from build123d import *

# Parameters (mm, degrees)
PAD_DEPTH       = 25
SKETCH001_R     = 4.3
POCKET_DEPTH    = 20.501
SKETCH002_R     = 6.75
POCKET001_DEPTH = 15.501
FILLET_R        = 4
FILLET001_R     = 18


with BuildPart() as part:
    # Sketch → Pad (new body)
    with BuildSketch(Plane.XZ):
        with BuildLine():
            Line((40.4, -20.4), (72.5, -20.4))
            Line((72.5, -20.4), (72.5, -30.4))
            Line((26.4, -40.9), (72.5, -30.4))
            Line((-26.4, -40.9), (26.4, -40.9))
            Line((-72.5, -30.4), (-26.4, -40.9))
            Line((-72.5, -30.4), (-72.5, -20.4))
            Line((-72.5, -20.4), (-40.4, -20.4))
            Line((-40.4, -21.9), (-40.4, -20.4))
            ThreePointArc((-26.4, -35.9), (-30.500505, -26.000505), (-40.4, -21.9))
            Line((-26.4, -35.9), (26.4, -35.9))
            ThreePointArc((40.4, -21.9), (30.500505, -26.000505), (26.4, -35.9))
            Line((40.4, -21.9), (40.4, -20.4))
        make_face()
    extrude(amount=PAD_DEPTH)

    # Sketch001 (on Face8 of Pad) → Pocket (cut, through all)
    with BuildSketch(Plane(origin=(0, 0, -20.4), x_dir=(-1, 0, 0), z_dir=(0, 0, 1))):
        with Locations((-60, 12.5)):
            Circle(SKETCH001_R)
        with Locations((60, 12.5)):
            Circle(SKETCH001_R)
    extrude(amount=-POCKET_DEPTH, mode=Mode.SUBTRACT)

    # Sketch002 (on Face13 of Pocket) → Pocket001 (cut, through all)
    with BuildSketch(Plane(origin=(0, 0, -25.4), x_dir=(-1, 0, 0), z_dir=(0, 0, 1))):
        with Locations((-60, 12.5)):
            Circle(SKETCH002_R)
        with Locations((60, 12.5)):
            Circle(SKETCH002_R)
    extrude(amount=-POCKET001_DEPTH, mode=Mode.SUBTRACT)

    # Fillet
    fillet_edges = [part.edges().sort_by_distance(p)[0] for p in [
        (-72.5, -25, -25.4),
        (-72.5, 0, -25.4),
        (72.5, -25, -25.4),
        (72.5, 0, -25.4),
    ]]
    fillet(fillet_edges, radius=FILLET_R)

    # Fillet001
    fillet001_edges = [part.edges().sort_by_distance(p)[0] for p in [
        (-26.4, -12.5, -40.9),
        (26.4, -12.5, -40.9),
    ]]
    fillet(fillet001_edges, radius=FILLET001_R)


solid = part.part
Check sheet for the modelled part. Datum: model origin and axes. Units: mm. A direction names the side the tool comes from. Round coordinates to 2 decimals unless told otherwise and drop trailing zeros. Loops run counter-clockwise (first coordinate to the right, second up) from the corner with the lowest first, then second, coordinate; pieces in that order, holes last. Notation, with made-up numbers: M 27,-21.5 L 68,-21.5 A14 cw 68,-1.5 Z; hole C 76.25,28.25 d9. An arc over 180 degrees is marked long. One line per item, written item: value.
(1) Sectioned sample at B-B, the plane x = -60. Record the cut outline in (y, z), then the cut area to 3 significant figures.
Computed values:
outline: M -25,-33.25 L -19.25,-33.25 L -19.25,-25.4 L -16.8,-25.4 L -16.8,-20.4 L -25,-20.4 Z; M -8.2,-25.4 L -5.75,-25.4 L -5.75,-33.25 L 0,-33.25 L 0,-20.4 L -8.2,-20.4 Z
area: 172 mm^2
(2) Sectioned sample at C-C, the plane x = -20. Record the cut outline in (y, z).
Computed values:
outline: M -25,-40.9 L 0,-40.9 L 0,-35.9 L -25,-35.9 Z
(3) Sectioned sample at A-A, the plane y = -12.5. Count the separate pieces of the cut face and the enclosed holes in it, then the cut area to 3 significant figures.
Computed values:
separate pieces: 3
enclosed holes: 0
area: 1,250 mm^2
(4) Sectioned sample at D-D, the plane z = -38.5. Record the cut outline in (x, y), then the cut area to 3 significant figures.
Computed values:
outline: M -36.94,-25 L 36.94,-25 L 36.94,0 L -36.94,0 Z
area: 1,850 mm^2
(5) Depth check by flat-ended pin: pin 1 Ø2 at (x, y) = (-51.5, -12) entering from -Z; pin 2 Ø11 at (x, y) = (63, -13.5) entering from -Z; pin 3 Ø11 at (x, y) = (-58, -15.5) entering from -Z. Enter the tip coordinate at first touch or a pass-through.
Computed values:
pin 1: stops at z = -35.41
pin 2: stops at z = -32.77
pin 3: stops at z = -34.96
(6) Access from +Z, -Z, +X, -X, +Y, -Y to the whole of each face (thin tool, end or side, straight path). Record for faces 1 (the face through (56, -10, -20.4)), 2 (the face through (-60, -8, -25.4)), 3 (the face through (-30.4, -12.3, -26.1)).
Computed values:
face 1: +Z, +X, -X, +Y, -Y
face 2: -Z
face 3: +Z, +Y, -Y
(7) Thickness scan on line 1 (X direction, y = -12.5, z = -21.5); line 2 (Y direction, x = 60, z = -23.55); line 3 (X direction, y = -20, z = -21.75). Record the ranges inside material, lowest first.
Computed values:
line 1: x = -72.5 to -64.3, -55.7 to -40.4, 40.4 to 55.7, 64.3 to 72.5
line 2: y = -25 to -16.8, -8.2 to 0
line 3: x = -72.5 to -40.4, 40.4 to 72.5
